Build history of the part. All positions in model axes, mm. Face numbers are marked on the shaded views. A direction names the side the tool comes from. Coordinates: 2 decimals unless noted, no trailing zeros. Write each loop counter-clockwise with the first axis right and the second up, starting at its lowest first coordinate (ties: lowest second). Pieces come first, ordered by that corner, then holes.
from build123d import *

# Parameters (mm, degrees)
F1_DEPTH = 12
F2_R     = 2.5
F3_DEPTH = 83.331666624
F4_W     = 6
F4_H     = 12
F4_R     = 1.5
F5_DEPTH = 3
F6_DEPTH = 6.5712102501


with BuildPart() as f1:
    # F0 (on Top) → F1 (new body)
    with BuildSketch(Plane.XY):
        Polygon((-20, -5), (-20, 0), (0, 0), (0, -5), (5, -5), (5, 83.330666624), (0, 83.330666624), (-25, 0), (-25, -5), align=None)
        Polygon((1, 4), (-19.6238279597, 4), (1, 72.743893289), align=None, mode=Mode.SUBTRACT)
    extrude(amount=F1_DEPTH)

    # F2 (on face) → F3 (cut, through all)
    with BuildSketch(Plane.XZ):
        with Locations((-10, 6)):
            Circle(F2_R)
    extrude(amount=-F3_DEPTH, mode=Mode.SUBTRACT)

    # F4 (on face) → F5 (join)
    with BuildSketch(Plane(origin=(-22.9356586075, 6.8809177751, 0), x_dir=(-0.2873563218, -0.9578237543, 0), z_dir=(-0.9578237543, 0.2873563218, 0))):
        with Locations((-76.816091954, 6)):
            Rectangle(F4_W, F4_H)
        with Locations((-76.816091954, 6)):
            Circle(F4_R, mode=Mode.SUBTRACT)
        with Locations((-11.816091954, 6)):
            Rectangle(F4_W, F4_H)
        with Locations((-11.816091954, 6)):
            Circle(F4_R, mode=Mode.SUBTRACT)
    extrude(amount=F5_DEPTH)

    # F4 (on face) → F6 (cut, through all)
    with BuildSketch(Plane(origin=(-22.9356586075, 6.8809177751, 0), x_dir=(-0.2873563218, -0.9578237543, 0), z_dir=(-0.9578237543, 0.2873563218, 0))):
        with Locations((-76.816091954, 6)):
            Circle(F4_R)
        with Locations((-11.816091954, 6)):
            Circle(F4_R)
    extrude(amount=-F6_DEPTH, mode=Mode.SUBTRACT)


solid = f1.part
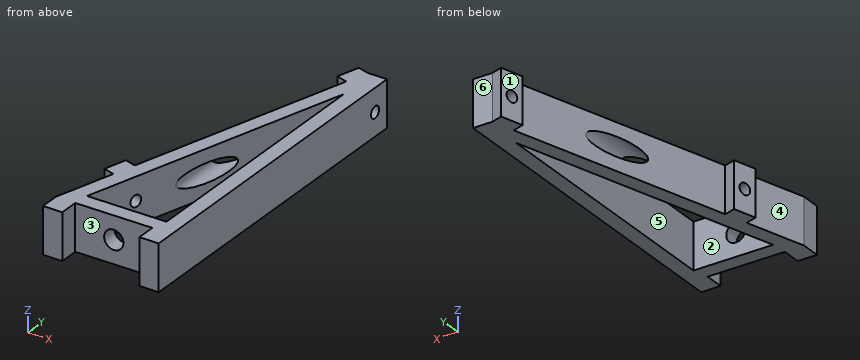
(1) Slice it at C-C, the plane x = -10. List the corners of the cut face in (y, z).
(2) Slice it at B-B, the plane y = 47. List the corners of the cut face in (x, z).
(3) Probe L1, parallel to Z at x = -10, y = 2.15; L2, parallel to X at y = 41.5, z = 11.75; L3, parallel to Y at x = 2, z = 6. List the from-to ranges inside material, lowest first.
(4) Slice it at A-A, the plane z = 10. List the corners of the cut face in (x, y), and give its area (3 significant figures).
(5) Flat gauge pins, fed straight in: P1, Ø6, axis at x = -10, z = 5.5, coming from the -Y side; P2, Ø3.5, axis at y = 40.5, z = 3, coming from the -X side; P3, Ø2.5, axis at x = 2, z = 5, coming from the +Y side. Where does each tip first touch, or does it go through?
(6) 3-axis set-ups, long thin cutter, end or side, ignore diameter. For the marked faces 4, 5 and 6: which of +Z, -Z, +X, -X, +Y, -Y reach the whole face in a straight line?
(7) Slice it at D-D, the plane z = 6. Give the number of separate pieces and of enclosed holes in the cut face, and give its area (3 significant figures).
(8) Two-plate mould, pull along Y, no slides. Class the marked faces 1, 2 and 3: pulls with the +Y half, pulls with the -Y half, needs draft (parallel to the pull), parting line crosses it, or undercut.
Results:
1. outline: (0, 0) - (4, 0) - (4, 3.5) - (0, 3.5) - close; (0, 8.5) - (4, 8.5) - (4, 12) - (0, 12) - close; (36.08, 0) - (50, 0) - (50, 3.5) - (36.08, 3.5) - close; (36.08, 8.5) - (50, 8.5) - (50, 12) - (36.08, 12) - close
2. outline: (-10.9, 0) - (-6.72, 0) - (-6.72, 12) - (-10.9, 12) - (-10.9, 8.33) arc R2.5 cw (long way) to (-10.9, 3.67) - close; (1, 0) - (5, 0) - (5, 12) - (1, 12) - close
3. L1: z = 0 to 3.5, 8.5 to 12
3. L2: x = -12.55 to -8.37, 1 to 5
3. L3: y = -5 to 78.03, 81.16 to 83.33
4. outline: (-25, -5) - (-20, -5) - (-20, 0) - (0, 0) - (0, -5) - (5, -5) - (5, 83.33) - (0, 83.33) - (-2.87, 84.19) - (-4.6, 78.45) - (-1.72, 77.58) - (-18.68, 21.07) - (-21.55, 21.93) - (-23.28, 16.19) - (-20.4, 15.33) - (-25, 0) - close; hole (-19.62, 4) - (1, 4) - (1, 72.74) - close
4. area: 835 mm2
5. P1: stops at y = 0
5. P2: stops at x = -13.37
5. P3: stops at y = 83.33
6. face 4: +Z, -Z, -X
6. face 5: +Z, -Z
6. face 6: +Z, -Z, +X, +Y
7. separate pieces: 4
7. enclosed holes: 0
7. area: 697 mm2
8. face 1: pulls with the +Y half
8. face 2: undercut
8. face 3: pulls with the -Y half
